Source: CAD feature listing. Evaluate the final solid. Frame: model axes, mm. A direction names the side the tool comes from. Coordinates: 2 decimals unless noted, no trailing zeros. Order: outer loops, then holes, each group sorted by start corner. A loop starts at its lowest first (then second) coordinate and runs counter-clockwise, first axis right, second up.
```python
from build123d import *

# Parameters (mm, degrees)
ISO4762_HEAD_SKETCH_R                   = 1.9
ISO4762_HEAD_DEPTH                      = 2
THREAD_MAJOR_DIAMETER_ENVELOPE_START    = -4
THREAD_MAJOR_DIAMETER_ENVELOPE_SKETCH_R = 1
THREAD_MAJOR_DIAMETER_ENVELOPE_DEPTH    = 4
HEX_SOCKET_START                        = 0.97
HEX_SOCKET_DEPTH                        = 1.03


with BuildPart() as part:
    # ISO4762_head_Sketch → ISO4762_head (new body)
    with BuildSketch(Plane.XY):
        Circle(ISO4762_HEAD_SKETCH_R)
    extrude(amount=ISO4762_HEAD_DEPTH)

    # Thread_major_diameter_envelope_Sketch → Thread_major_diameter_envelope (add)
    with BuildSketch(Plane.XY.offset(THREAD_MAJOR_DIAMETER_ENVELOPE_START)):
        Circle(THREAD_MAJOR_DIAMETER_ENVELOPE_SKETCH_R)
    extrude(amount=THREAD_MAJOR_DIAMETER_ENVELOPE_DEPTH)

    # Hex_socket_Sketch → Hex_socket (cut)
    with BuildSketch(Plane.XY.offset(HEX_SOCKET_START)):
        Polygon((0.866025404, 0), (0.433012702, 0.75), (-0.433012702, 0.75), (-0.866025404, 0), (-0.433012702, -0.75), (0.433012702, -0.75), align=None)
    extrude(amount=HEX_SOCKET_DEPTH, mode=Mode.SUBTRACT)


solid = part.part
```
1. Section query C-C on y = 1.75. Return loops of the section in (x, z), plus the area to 3 significant figures.
Findings:
outline: (-0.74, 0) - (0.74, 0) - (0.74, 2) - (-0.74, 2) - close
area: 2.96 mm2
2. Ray query, line 1 (Z direction, x = -0.15, y = -1.5); line 2 (X direction, y = -0.05, z = -3.5); line 3 (X direction, y = -0.35, z = 1.7). Return the intervals inside material, ascending.
Findings:
line 1: z = 0 to 2
line 2: x = -1 to 1
line 3: x = -1.87 to -0.66, 0.66 to 1.87
3. Pin query (flat end, axial travel): P1, Ø1.5, axis at y = 1, z = -1.5, coming from the +X side. Return the tip coordinate at first contact, or that it passes through.
Findings:
P1: stops at x = 0.97
4. Section query D-D on x = 0.65. Return loops of the section in (y, z).
Findings:
outline: (-1.79, 0) - (-0.76, 0) - (-0.76, -4) - (0.76, -4) - (0.76, 0) - (1.79, 0) - (1.79, 2) - (0.37, 2) - (0.37, 0.97) - (-0.37, 0.97) - (-0.37, 2) - (-1.79, 2) - close
5. Section query A-A on x = 0. Return loops of the section in (y, z).
Findings:
outline: (-1.9, 0) - (-1, 0) - (-1, -4) - (1, -4) - (1, 0) - (1.9, 0) - (1.9, 2) - (0.75, 2) - (0.75, 0.97) - (-0.75, 0.97) - (-0.75, 2) - (-1.9, 2) - close
6. Section query B-B on z = 0.8. Return loops of the section in (x, y), plus the area to 3 significant figures.
Findings:
outline: circle Ø3.8 at (0, 0)
area: 11.3 mm2
7. Draft query along Y for faces 4 (the face through (0, -1, -2)), 5 (the face through (0, -1, 2)), 6 (the face through (0, 0, 0.97)). Return one class per face: released by +Y, released by -Y, zero draft, split by the parting line, or undercut.
Findings:
face 4: split by the parting line
face 5: zero draft
face 6: undercut
8. Access query for faces 1 (the face through (1, -1, 0)), 2 (the face through (0, -0.75, 1.5)), 3 (the face through (0, 0, -4)). Directions: +Z, -Z, +X, -X, +Y, -Y. A direction counts if a zero-diameter tool reaches every point of the face in a straight line with its end or side. Return the directions, or none.
Findings:
face 1: -Z
face 2: +Z
face 3: -Z, +X, -X, +Y, -Y
